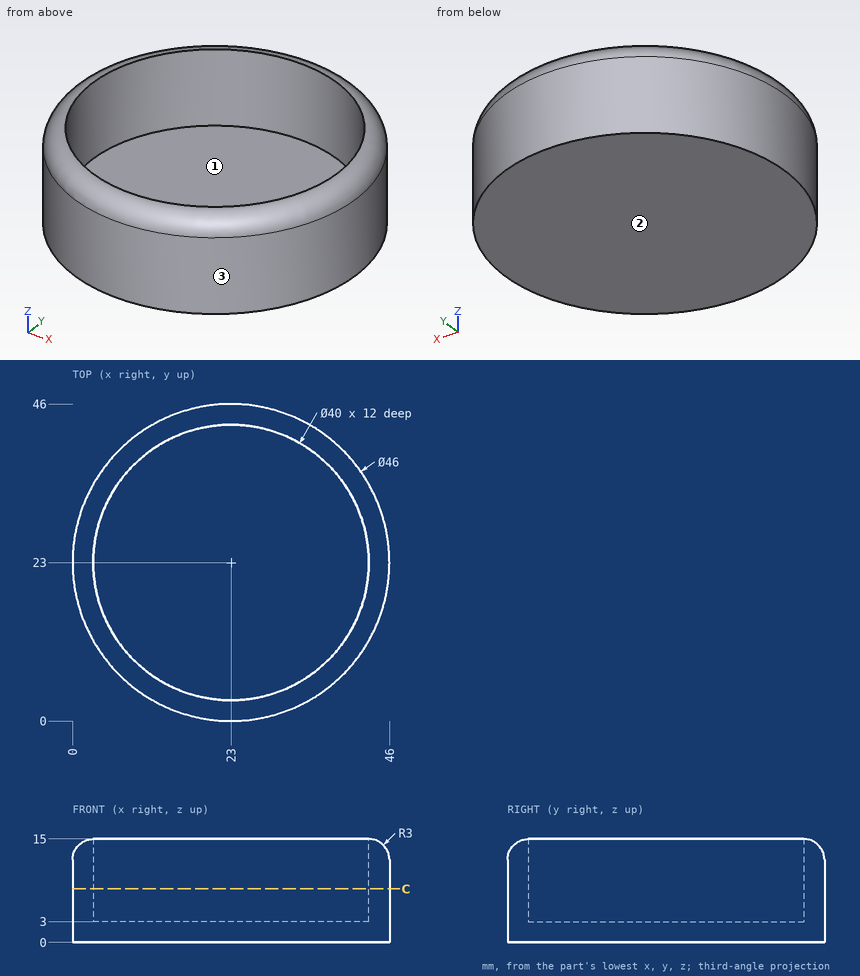
Can you work these out from the drawing? Everything is in mm from the part's minimum corner. Coordinates: 2 decimals unless noted, no trailing zeros. Loops run counter-clockwise (first coordinate to the right, second up) from the corner with the lowest first, then second, coordinate; pieces in that order, holes last.
1. I need wall thicknesses on L1, parallel to Y at x = 23, z = 11.5; L2, parallel to Z at x = 12, y = 28.5; L3, parallel to X at y = 31, z = 9.5. Which ranges of each line are inside material? Lowest first, please.
2. Imagine slicing it at C-C, the plane z = 7.75. Please give me the cut outline in (x, y), and give its area (3 significant figures).
3. If we mould it in two halves opening along X, with no side actions, what happens to the marked faces 1, 2 and 3? For each: pulls with the +X half, pulls with the -X half, needs draft (parallel to the pull), parting line crosses it, or undercut.
4. For P1, Ø2, axis at x = 12.5, y = 33.5, coming from the +Z side; P2, Ø4, axis at x = 15, y = 21.5, coming from the -Z side; P3, Ø5, axis at x = 41.5, z = 9.5, coming from the +Y side; P4, Ø5, axis at y = 28.5, z = 2.5, coming from the +X side, each with a flat end and sliding along its axis, tell me the tip position at first contact or that it passes through.
Taken from the geometry:
1. L1: y = 0 to 3, 43 to 46
1. L2: z = 0 to 3
1. L3: x = 1.44 to 4.67, 41.33 to 44.56
2. outline: circle Ø46 at (23, 23); hole circle Ø40 at (23, 23)
2. area: 405 mm2
3. face 1: undercut
3. face 2: needs draft
3. face 3: parting line crosses it
4. P1: stops at z = 3
4. P2: stops at z = 0
4. P3: stops at y = 39.52
4. P4: stops at x = 45.8
